Autodesk Inventor part; units mm, degrees
ref_plane "YZ Plane" through (0, 0, 0) normal (1, 0, 0) x (0, 1, 0)
ref_plane "XZ Plane" through (0, 0, 0) normal (0, 1, 0) x (-1, 0, 0)
ref_plane "XY Plane" through (0, 0, 0) normal (0, 0, 1) x (1, 0, 0)
sketch "Sketch1" plane through (0, 0, 0) normal (0, 0, 1) x (1, 0, 0)
  line L0 (0, 0) -> (21, 0)
  line L1 (21, 0) -> (21, 11)
  line L2 (21, 11) -> (0, 11)
  line L3 (0, 11) -> (0, 0)
  dimension "d0" = 21
  dimension "d1" = 11
extrude "Extrusion1" add sketch "Sketch1" along normal blind 10
sketch "Sketch2" plane through (0, 0, 10) normal (0, 0, 1) x (1, 0, 0)
  line L0 (0, 0) -> (21, 0)
  arc A0 (4.3181, 0) -> (5.25, 3.5) centre (4.3181, 1.8741) ccw
  arc A1 (6.1819, 7) -> (5.25, 3.5) centre (6.1819, 5.1259) ccw
  arc A2 (15.75, 3.5) -> (16.6819, 0) centre (16.6819, 1.8741) ccw
  arc A3 (15.75, 3.5) -> (14.8181, 7) centre (14.8181, 5.1259) ccw
  line L1 (6.1819, 7) -> (14.8181, 7)
  line L2 (21, 11) -> (0, 11)
  line L3 (4.3181, 1.8741) -> (6.1819, 5.1259) construction
  line L4 (16.6819, 1.8741) -> (14.8181, 5.1259) construction
  line L5 (0, 11) -> (0, 0) construction
  line L6 (21, 0) -> (21, 11) construction
  point P0 (10.5, 7)
  point P1 (15.75, 3.5)
  dimension "d7" = 10.5
  dimension "d9" = 7
  dimension "d13" = 10.5
extrude "Extrusion2" cut sketch "Sketch2" against normal through all
sketch "Sketch3" plane through (0, 0, 10) normal (0, 0, 1) x (1, 0, 0)
  line L0 (21, 11) -> (0, 11)
  line L1 (14.8181, 7) -> (6.1819, 7)
  arc A0 (6.6147, 7) -> (10, 10) centre (6.6147, 10.41) ccw
  arc A1 (11, 10) -> (14.3853, 7) centre (14.3853, 10.41) ccw
  line L2 (10, 10) -> (11, 10)
  line L3 (6.1819, 7) -> (14.8181, 7)
  line L4 (10.5, 10) -> (10.5, 11) construction
  point P0 (0, 0)
  dimension "d15" = 1
  dimension "d16" = 1
extrude "Extrusion3" cut sketch "Sketch3" against normal through all
pattern_linear "Rectangular Pattern1" count 6 spacing 21 along (1, 0, 0)
sketch "Sketch4" plane through (0, 0, 10) normal (0, 0, 1) x (1, 0, 0)
  line L0 (115, 10) -> (116, 10)
  line L1 (115, 10) -> (115, 11)
  line L2 (126, 11) -> (0, 11)
  line L3 (121.6819, 0) -> (126, 0)
  line L4 (121.6819, 0) -> (126, 0)
  line L5 (126, 0) -> (126, 11)
  line L6 (126, 0) -> (126, 11)
  line L7 (126, 11) -> (115, 11)
  arc A0 (116, 10) -> (119.3853, 7) centre (119.3853, 10.41) ccw
  line L8 (115, 10) -> (116, 10)
  line L9 (119.3853, 7) -> (119.8181, 7)
  arc A1 (116, 10) -> (119.3853, 7) centre (119.3853, 10.41) ccw
  arc A2 (120.75, 3.5) -> (119.8181, 7) centre (119.8181, 5.1259) ccw
  line L10 (119.3853, 7) -> (119.8181, 7)
  arc A3 (120.75, 3.5) -> (119.8181, 7) centre (119.8181, 5.1259) ccw
  arc A4 (120.75, 3.5) -> (121.6819, 0) centre (121.6819, 1.8741) ccw
  arc A5 (120.75, 3.5) -> (121.6819, 0) centre (121.6819, 1.8741) ccw
  line L11 (32, 10) -> (31, 10)
  line L12 (31, 10) -> (31, 11)
  line L13 (31, 10) -> (31, 0)
  line L14 (31, 0) -> (126, 0)
  line L15 (126, 11) -> (31, 11)
  arc A6 (11, 10) -> (14.3853, 7) centre (14.3853, 10.41) ccw
  line L16 (11, 10) -> (10.8789, 11)
  line L17 (10.8789, 11) -> (0, 11)
  line L18 (0, 11) -> (0, 0)
  line L19 (0, 0) -> (11, 0)
  line L20 (11, 0) -> (11, 10)
  point P0 (11, 11)
extrude "Extrusion4" cut sketch "Sketch4" against normal through all
sketch "Sketch5" plane through (0, 0, 10) normal (0, 0, 1) x (1, 0, 0)
  line L0 (31, 11) -> (10.8789, 11)
  line L1 (15.75, 3.5) -> (12.112, 9.8474) construction
  arc A0 (15.75, 3.5) -> (16.6819, 0) centre (16.6819, 1.8741) ccw construction
  line L2 (11.7707, 1.2193) -> (15.75, 3.5) construction
  arc A1 (15.75, 3.5) -> (14.8181, 7) centre (14.8181, 5.1259) ccw construction
  line L3 (15.75, 3.5) -> (19.849, 5.8494) construction
  arc A2 (25.3181, 0) -> (26.25, 3.5) centre (25.3181, 1.8741) ccw construction
  line L4 (26.25, 3.5) -> (29.888, 9.8474) construction
  line L5 (23.4673, 5.0949) -> (26.25, 3.5) construction
  line L6 (26.25, 3.5) -> (28.9514, 1.9517) construction
  arc A3 (25.3181, 0) -> (26.25, 3.5) centre (25.3181, 1.8741) ccw construction
  line L7 (12.112, 9.8474) -> (8.7461, 15.7199) construction
  line L8 (29.888, 9.8474) -> (33.5756, 16.2813) construction
  line L9 (21.2593, -5.2075) -> (20.7407, -6.1122) construction
  arc A4 (15.75, 3.5) -> (16.6819, 0) centre (16.6819, 1.8741) ccw construction
  arc A5 (15.75, 3.5) -> (14.8181, 7) centre (14.8181, 5.1259) ccw construction
  arc A6 (27.1819, 7) -> (26.25, 3.5) centre (27.1819, 5.1259) ccw construction
properties part number "Zipperteethv4.2"
Work out the finished part from the listing and answer in its coordinate system (mm). Coordinates: 2 decimals unless noted, no trailing zeros. Write each loop counter-clockwise with the first axis right and the second up, starting at its lowest first coordinate (ties: lowest second). Pieces come first, ordered by that corner, then holes. Notation, with made-up numbers: M 36,-20 L 90,-20 A11 cw 90,-11 Z; hole C 8.5,10 d7. An arc over 180 degrees is marked long. Write item = value, one per line.
1. The part is cut by section C-C (x = 29). Determine the outline of the cut face in (y, z), then the cut area to 3 significant figures.
Solution:
outline = M 7.29,0 L 11,0 L 11,10 L 7.29,10 Z
area = 37.1 mm2
2. The part is cut by section A-A (z = 9.75). Determine the outline of the cut face in (x, y).
Solution:
outline = M 10.88,11 L 11,10 A3.41 ccw 14.39,7 L 14.82,7 A1.87 cw 15.75,3.5 A1.87 ccw 16.68,0 L 25.32,0 A1.87 ccw 26.25,3.5 A1.87 cw 27.18,7 L 27.61,7 A3.41 ccw 31,10 L 31,11 Z
3. Straight lines are drawn through the part: line 1 (X direction, y = 1.75, z = 9.75); line 2 (Y direction, x = 27.25, z = 2.75); line 3 (X direction, y = 5, z = 3.75). For each, find the intervals that lie inside material, in ascending order. Write a range as from..to.
Solution:
line_1 = 14.81..27.19
line_2 = 7..11
line_3 = 16.69..25.31
4. The part is cut by section B-B (y = 9). Determine the outline of the cut face in (x, z), then the cut area to 3 significant figures.
Solution:
outline = M 11.28,0 L 30.72,0 L 30.72,10 L 11.28,10 Z
area = 194 mm2
